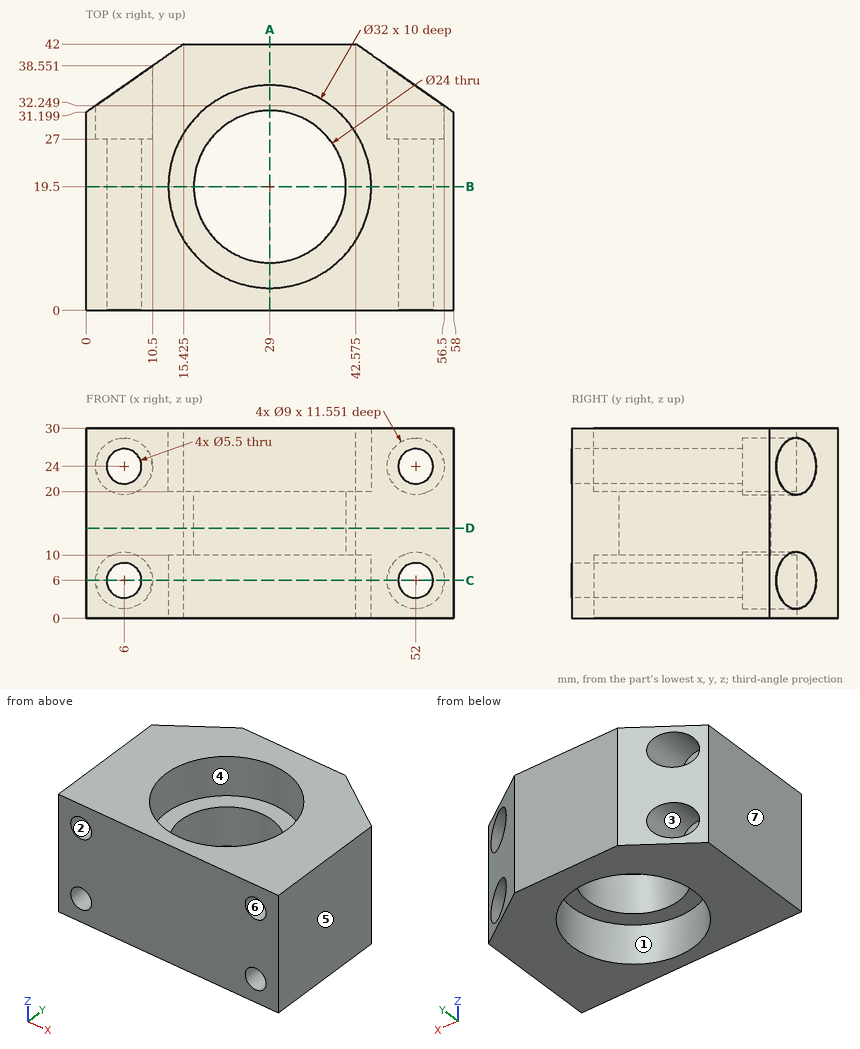
Can you work these out from the drawing? Everything is in mm from the part's minimum corner. A direction names the side the tool comes from. Coordinates: 2 decimals unless noted, no trailing zeros. Loops run counter-clockwise (first coordinate to the right, second up) from the corner with the lowest first, then second, coordinate; pieces in that order, holes last.
1) Will these pins go through, and if not, where does the flat tip stop? pin 1 Ø16 at (x, y) = (25, 16.5) entering from +Z; pin 2 Ø3.5 at (x, z) = (52, 24) entering from +Y; pin 3 Ø10 at (x, z) = (5, 5.5) entering from +Y (1 decimal); pin 4 Ø14.5 at (x, z) = (6, 6) entering from +Y.
Reported:
pin 1: stops at z = 20
pin 2: passes through
pin 3: stops at y = 37.7
pin 4: stops at y = 40.48
2) Imagine slicing it at D-D (z = 14.25). List the corners of the cut face in (x, y) for me (1 decimal), and give its area (3 significant figures).
Reported:
outline: (0, 0) - (58, 0) - (58, 31.2) - (42.6, 42) - (15.4, 42) - (0, 31.2) - close; hole circle Ø24 at (29, 19.5)
area: 1,820 mm2
3) Which directions (+Z, -Z, +X, -X, +Y, -Y) give clear straight access to the entire face, cutting with the end or side of a thin tool? Please do the marked faces 1, 2 and 3.
Reported:
face 1: -Z
face 2: +Y, -Y
face 3: +Y
4) Please list where these lines run through material, in increasing order: line 1 along Z through (x, y) = (52, 33.5); line 2 along Z through (x, y) = (6, 18.25); line 3 along Y through (x, z) = (29, 4.25).
Reported:
line 1: z = 0 to 1.5, 10.5 to 19.5, 28.5 to 30
line 2: z = 0 to 3.25, 8.75 to 21.25, 26.75 to 30
line 3: y = 0 to 3.5, 35.5 to 42
5) Imagine slicing it at C-C (z = 6). State how many separate pieces and enclosed holes the cut face has, and give its area (3 significant figures).
Reported:
separate pieces: 3
enclosed holes: 1
area: 1,020 mm2
6) Imagine slicing it at A-A (x = 29). List the corners of the cut face in (y, z) for me.
Reported:
outline: (0, 0) - (3.5, 0) - (3.5, 10) - (7.5, 10) - (7.5, 20) - (3.5, 20) - (3.5, 30) - (0, 30) - close; (31.5, 10) - (35.5, 10) - (35.5, 0) - (42, 0) - (42, 30) - (35.5, 30) - (35.5, 20) - (31.5, 20) - close
7) Imagine slicing it at B-B (y = 19.5). List the corners of the cut face in (x, z) for me.
Reported:
outline: (0, 0) - (13, 0) - (13, 10) - (17, 10) - (17, 20) - (13, 20) - (13, 30) - (0, 30) - close; (41, 10) - (45, 10) - (45, 0) - (58, 0) - (58, 30) - (45, 30) - (45, 20) - (41, 20) - close; hole circle Ø5.5 at (6, 6); hole circle Ø5.5 at (6, 24); hole circle Ø5.5 at (52, 6); hole circle Ø5.5 at (52, 24)
8) Thinking about a two-plate mould opening in X: for the marked faces 4, 5, 6 and 7, which applies, released by +X, released by -X, zero draft, split by the parting line, or undercut?
Reported:
face 4: undercut
face 5: released by +X
face 6: undercut
face 7: released by -X
